Here's how the part is built. I have some questions about the finished solid (model axes, mm). A direction names the side the tool comes from. Round coordinates to 2 decimals unless told otherwise and drop trailing zeros. Loops run counter-clockwise (first coordinate to the right, second up) from the corner with the lowest first, then second, coordinate; pieces in that order, holes last. Notation, with made-up numbers: (12.25, -14.5) -> (29.25, -14.5) arc R18 ccw to (29.25, 15.5) -> close; hole circle Ø2 at (72.25, -18.5). An arc over 180 degrees is marked (long way). Use CSV: the item, a comma, the result in double quotes. Start each with the question number.
from build123d import *

# Parameters (mm, degrees)
BOSS_EXTRUDE1_DEPTH = 2.5
SKETCH2_R           = 3.5
BOSS_EXTRUDE2_DEPTH = 2.5
FILLET1_R           = 6.35
FILLET2_R           = 6.35
FILLET3_R           = 3
BOSS_EXTRUDE3_DEPTH = 5
CUT_EXTRUDE1_REACH  = 217.584
SKETCH3_4_R         = 3.5


with BuildPart() as part:
    # Sketch1 → Boss-Extrude1 (new, symmetric)
    with BuildSketch(Plane(origin=(0, 0, 0), x_dir=(1, 0, 0), z_dir=(0, 1, 0))):
        Polygon((63.5, 152.4), (127, 152.4), (127, -152.4), (-127, -152.4), (-127, 152.4), (-63.5, 152.4), (-50.8, 139.7), (50.8, 139.7), align=None)
    extrude(amount=BOSS_EXTRUDE1_DEPTH, both=True)

    # Sketch2 → Boss-Extrude2 (add, symmetric)
    # profile 1 of 2: a face of its own
    with BuildSketch(Plane(origin=(0, 0, 0), x_dir=(1, 0, 0), z_dir=(0, 1, 0))):
        Polygon((127, 152.4), (152.4, 152.4), (152.4, 127), (146.05, 101.6), (146.05, -101.6), (152.4, -127), (152.4, -152.4), (127, -152.4), align=None)
        with Locations(Location((137.4, 139.7, 0), (0, 0, 270))):
            Circle(SKETCH2_R, mode=Mode.SUBTRACT)
        with Locations(Location((137.4, -139.7, 0), (0, 0, 270))):
            Circle(SKETCH2_R, mode=Mode.SUBTRACT)
    # profile 2 of 2: a face of its own
    with BuildSketch(Plane(origin=(0, 0, 0), x_dir=(1, 0, 0), z_dir=(0, 1, 0))):
        Polygon((-127, 152.4), (-152.4, 152.4), (-152.4, 127), (-146.05, 101.6), (-146.05, -101.6), (-152.4, -127), (-152.4, -152.4), (-127, -152.4), align=None)
        with Locations(Location((-137.4, -139.7, 0), (0, 0, 90))):
            Circle(SKETCH2_R, mode=Mode.SUBTRACT)
        with Locations(Location((-137.4, 139.7, 0), (0, 0, 90))):
            Circle(SKETCH2_R, mode=Mode.SUBTRACT)
    extrude(amount=BOSS_EXTRUDE2_DEPTH, both=True)

    # Fillet1
    fillet1_edges = [part.edges().sort_by_distance(p)[0] for p in [
        (152.4, 0, 152.4),
        (152.4, 0, -152.4),
        (-152.4, 0, -152.4),
        (-152.4, 0, 152.4),
    ]]
    fillet(fillet1_edges, radius=FILLET1_R)

    # Fillet2
    fillet2_edges = [part.edges().sort_by_distance(p)[0] for p in [
        (-63.5, 0, -152.4),
        (-50.8, 0, -139.7),
        (50.8, 0, -139.7),
        (63.5, 0, -152.4),
    ]]
    fillet(fillet2_edges, radius=FILLET2_R)

    # Fillet3
    fillet3_edges = [part.edges().sort_by_distance(p)[0] for p in [
        (152.4, 0, 127),
        (146.05, 0, 101.6),
        (146.05, 0, -101.6),
        (152.4, 0, -127),
        (-152.4, 0, -127),
        (-146.05, 0, -101.6),
        (-146.05, 0, 101.6),
        (-152.4, 0, 127),
    ]]
    fillet(fillet3_edges, radius=FILLET3_R)

    # Sketch3 → Boss-Extrude3 (add)
    with BuildSketch(Plane(origin=(0, 2.5, 0), x_dir=(1, 0, 0), z_dir=(0, 1, 0))):
        Polygon((-146.05, 19.05), (-152.4, 12.7), (-152.4, -12.7), (-146.05, -19.05), align=None)
        Polygon((152.4, -12.7), (152.4, 12.7), (146.05, 19.05), (146.05, -19.05), align=None)
    extrude(amount=-BOSS_EXTRUDE3_DEPTH)

    # Sketch3<4> → Cut-Extrude1 (cut, up to next)
    with BuildSketch(Plane(origin=(0, 2.5, 0), x_dir=(1, 0, 0), z_dir=(0, 1, 0)), mode=Mode.PRIVATE) as cut_extrude1_sk1:
        with Locations(Location((-137.4, 0, 0), (0, 0, 270))):
            Circle(SKETCH3_4_R)
    cut_extrude1_tool1 = extrude(cut_extrude1_sk1.sketch, amount=-CUT_EXTRUDE1_REACH, mode=Mode.PRIVATE) & part.part
    # Sketch3<4> → Cut-Extrude1 (cut, up to next)
    with BuildSketch(Plane(origin=(0, 2.5, 0), x_dir=(1, 0, 0), z_dir=(0, 1, 0)), mode=Mode.PRIVATE) as cut_extrude1_sk2:
        with Locations(Location((137.4, 0, 0), (0, 0, 270))):
            Circle(SKETCH3_4_R)
    cut_extrude1_tool2 = extrude(cut_extrude1_sk2.sketch, amount=-CUT_EXTRUDE1_REACH, mode=Mode.PRIVATE) & part.part
    add(cut_extrude1_tool1.solids().sort_by_distance((-137.4, 2.5, 0))[0], mode=Mode.SUBTRACT)
    add(cut_extrude1_tool2.solids().sort_by_distance((137.4, 2.5, 0))[0], mode=Mode.SUBTRACT)


solid = part.part
Q1. I want a section at D-D, the plane z = -53. List the corners of the cut face in (x, y) for me.
Q2. I want a section at C-C, the plane y = 1.15. Count the separate pieces of the cut face and the enclosed holes in it, then the cut area to 3 significant figures.
Q3. Will these pins go through, and if not, where does the flat tip stop? pin 1 Ø1.5 at (y, z) = (-1.5, 63.5) entering from +X; pin 2 Ø2.5 at (y, z) = (-1, -61) entering from -X; pin 3 Ø5.5 at (x, z) = (137.4, -139.7) entering from +Y; pin 4 Ø3 at (y, z) = (-1.5, -101) entering from +X (3 decimals).
Q4. I want a section at B-B, the plane x = -137.4. List the corners of the cut face in (y, z) for me.
Q5. If we mould it in two halves opening along Z, with no side actions, what happens to faces 1 (the flat face through (-2, 2.5, -2)), 2 (the flat face through (-57.2, 0, -146.1)), 3 (the cylindrical face through (133.983, 0.035, -0.759))? For each: pulls with the +Z half, pulls with the -Z half, needs draft (parallel to the pull), parting line crosses it, or undercut.
Q6. I need wall thicknesses on line 1 along X through (y, z) = (1.3, 139.7); line 2 along Z through (x, y) = (-137.4, 1.45); line 3 along X through (y, z) = (1.7, 1). Which ranges of each line are inside material? Lowest first, please.
Q7. For faces 4 (the cylindrical face through (-133.983, -0.035, -138.941)), 5 (the flat face through (57.1, 0, -146)), which set-ups out of +Z, -Z, +X, -X, +Y, -Y let a thin tool reach every point of the face, with its end or its side?
Q8. I want a section at A-A, the plane z = 0. List the corners of the cut face in (x, y) for me, then the cut area to 3 significant figures.
Values found:
1,outline,"(-146.05, -2.5) -> (146.05, -2.5) -> (146.05, 2.5) -> (-146.05, 2.5) -> close"
2,separate pieces,"1"
2,enclosed holes,"6"
2,area,"88,700 mm2"
3,pin 1,"x = 146.05"
3,pin 2,"x = -146.05"
3,pin 3,"through"
3,pin 4,"x = 146.275"
4,outline,"(-2.5, -152.4) -> (2.5, -152.4) -> (2.5, -143.2) -> (-2.5, -143.2) -> close; (-2.5, -136.2) -> (2.5, -136.2) -> (2.5, -3.5) -> (-2.5, -3.5) -> close; (-2.5, 3.5) -> (2.5, 3.5) -> (2.5, 136.2) -> (-2.5, 136.2) -> close; (-2.5, 143.2) -> (2.5, 143.2) -> (2.5, 152.4) -> (-2.5, 152.4) -> close"
5,face 1,"needs draft"
5,face 2,"pulls with the -Z half"
5,face 3,"undercut"
6,line 1,"-152.4 to -140.9, -133.9 to 133.9, 140.9 to 152.4"
6,line 2,"-152.4 to -143.2, -136.2 to -3.5, 3.5 to 136.2, 143.2 to 152.4"
6,line 3,"-152.4 to -140.75, -134.05 to 134.05, 140.75 to 152.4"
7,face 4,"+Y, -Y"
7,face 5,"-Z, +Y, -Y"
8,outline,"(-152.4, -2.5) -> (-140.9, -2.5) -> (-140.9, 2.5) -> (-152.4, 2.5) -> close; (-133.9, -2.5) -> (133.9, -2.5) -> (133.9, 2.5) -> (-133.9, 2.5) -> close; (140.9, -2.5) -> (152.4, -2.5) -> (152.4, 2.5) -> (140.9, 2.5) -> close"
8,area,"1,450 mm2"
